```python
from build123d import *

# Parameters (mm, degrees)
SKETCH_W         = 114
SKETCH_H         = 30
PAD_DEPTH        = 15
POCKET_DEPTH     = 30.001
POCKET001_DEPTH  = 12.5
HOLE_D           = 3
HOLE_CBORE_D     = 6
HOLE_CBORE_DEPTH = 3.5
FILLET_R         = 2.5


with BuildPart() as part:
    # Sketch → Pad (new body)
    with BuildSketch(Plane.XY):
        Rectangle(SKETCH_W, SKETCH_H)
    extrude(amount=PAD_DEPTH)

    # Sketch001 (on Face2 of Pad) → Pocket (cut, through all)
    with BuildSketch(Plane.XZ.offset(15)):
        with BuildLine():
            ThreePointArc((-36, 15), (-32.719596, 7.080404), (-24.8, 3.8))
            Line((-24.8, 3.8), (24.8, 3.8))
            ThreePointArc((24.8, 3.8), (32.719596, 7.080404), (36, 15))
            Line((-36, 15), (36, 15))
        make_face()
    extrude(amount=-POCKET_DEPTH, mode=Mode.SUBTRACT)

    # Sketch002 (on DatumPlane) → Pocket001 (cut, symmetric)
    with BuildSketch(Plane.XZ):
        with BuildLine():
            ThreePointArc((-36.754336, 13.954131), (-33.285281, 6.514719), (-25.845869, 3.045664))
            Line((-24.8, 15), (-25.845869, 3.045664))
            Line((-36.754336, 13.954131), (-24.8, 15))
        make_face()
        with BuildLine():
            ThreePointArc((25.845869, 3.045664), (33.285281, 6.514719), (36.754336, 13.954131))
            Line((36.754336, 13.954131), (24.8, 15))
            Line((25.845869, 3.045664), (24.8, 15))
        make_face()
    extrude(amount=POCKET001_DEPTH, both=True, mode=Mode.SUBTRACT)

    # Hole (through all)
    with Locations(Plane(origin=(0, 0, 0), x_dir=(1, 0, 0), z_dir=(0, 0, -1))):
        with Locations((-46.5, 0), (46.5, 0)):
            CounterBoreHole(HOLE_D / 2, HOLE_CBORE_D / 2, HOLE_CBORE_DEPTH)

    # Fillet
    fillet_edges = [part.edges().sort_by_distance(p)[0] for p in [
        (-57, -15, 7.5),
        (57, -15, 7.5),
        (57, 0, 0),
        (-57, 0, 0),
        (0, -15, 0),
    ]]
    fillet(fillet_edges, radius=FILLET_R)


solid = part.part
```
Can you work these out from the model? Positions are in its coordinate system, mm. A direction names the side the tool comes from. Coordinates: 2 decimals unless noted, no trailing zeros. Order: outer loops, then holes, each group sorted by start corner. A loop starts at its lowest first (then second) coordinate and runs counter-clockwise, first axis right, second up.
1. Thinking about a two-plate mould opening in X: for faces 1 (the face through (-45, 0, 9)), 2 (the face through (-44, 0, 15)), 3 (the face through (-56.287, -14.248, 8.838)), which applies, +X half, -X half, draft (parallel to the pull), parting line (faces both ways), or undercut?
2. If we section it at B-B (x = -46.5): Please give me the cut outline in (y, z).
3. I'm going to push flat-ended pins straight in: pin 1 (9 mm diameter, centred on x = 29.5, z = 9, fed in from +Y); pin 2 (12 mm diameter, centred on x = -8.5, y = -1.5, fed in from +Z); pin 3 (5 mm diameter, centred on x = -46.5, y = 0, fed in from -Z). Where does each tip first touch, or does it pass through?
4. If we section it at A-A (y = 0): Give the number of separate pieces and of enclosed holes in the cut face, then the cut area to 3 significant figures.
5. I need wall thicknesses on line 1 (X direction, y = -5.25, z = 13.75); line 2 (Y direction, x = 46.5, z = 10.5); line 3 (Z direction, x = 13, y = -5.5). Which ranges of each line are inside material? Lowest first, please.
6. If we section it at D-D (y = 4.25): Please give me the cut outline in (x, z).
7. For faces 4 (the face through (-1, 1, 0)), 5 (the face through (-1, 15, 2)), 6 (the face through (-33, -12.5, 7)), 7 (the face through (0, 0, 3.8)), 8 (the face through (-48, 1, 3.5)), which set-ups out of +Z, -Z, +X, -X, +Y, -Y let a thin tool reach every point of the face, with its end or its side?
8. If we section it at C-C (z = 9.25): Please give me the cut outline in (x, y), then the cut area to 3 significant figures.
Entries:
1. face 1: undercut
1. face 2: draft
1. face 3: -X half
2. outline: (-15, 2.5) arc R2.5 ccw to (-12.5, 0) - (-3, 0) - (-3, 3.5) - (-1.5, 3.5) - (-1.5, 15) - (-15, 15) - close; (1.5, 3.5) - (3, 3.5) - (3, 0) - (15, 0) - (15, 15) - (1.5, 15) - close
3. pin 1: stops at y = 15
3. pin 2: stops at z = 3.8
3. pin 3: stops at z = 3.5
4. separate pieces: 3
4. enclosed holes: 0
4. area: 818 mm2
5. line 1: x = -57 to -36.73, 36.73 to 57
5. line 2: y = -15 to -1.5, 1.5 to 15
5. line 3: z = 0 to 3.8
6. outline: (-57, 2.5) arc R2.5 ccw to (-54.5, 0) - (54.5, 0) arc R2.5 ccw to (57, 2.5) - (57, 15) - (36, 15) arc R11.2 cw to (35.96, 14.02) - (36.75, 13.95) arc R12 cw to (25.85, 3.05) - (25.78, 3.84) arc R11.2 cw to (24.8, 3.8) - (-24.8, 3.8) arc R11.2 cw to (-25.78, 3.84) - (-25.85, 3.05) arc R12 cw to (-36.75, 13.95) - (-35.96, 14.02) arc R11.2 cw to (-36, 15) - (-57, 15) - close
7. face 4: -Z, +X, -X, +Y, -Y
7. face 5: +Z, -Z, +X, -X, +Y
7. face 6: none
7. face 7: +Z, +Y, -Y
7. face 8: -Z
8. outline: (-57, -12.5) arc R2.5 ccw to (-54.5, -15) - (-34.41, -15) - (-34.41, -12.5) - (-35.33, -12.5) - (-35.33, 12.5) - (-34.41, 12.5) - (-34.41, 15) - (-57, 15) - close; (34.41, -15) - (54.5, -15) arc R2.5 ccw to (57, -12.5) - (57, 15) - (34.41, 15) - (34.41, 12.5) - (35.33, 12.5) - (35.33, -12.5) - (34.41, -12.5) - close; hole circle Ø3 at (-46.5, 0); hole circle Ø3 at (46.5, 0)
8. area: 1,290 mm2
